```python
from build123d import *

# Parameters (mm, degrees)
F0_W     = 61
F0_H     = 49.2
F1_DEPTH = 1
F2_D     = 3.5
F3_R     = 3.75
F4_DEPTH = 8
F3_R_2   = 6.25
F5_DEPTH = 5
F6_R     = 21
F7_DEPTH = 15
F8_R     = 6.25
F9_DEPTH = 7


with BuildPart() as f1:
    # F0 (on Top) → F1 (new body)
    with BuildSketch(Plane.XY):
        with Locations((30.5, 24.6)):
            Rectangle(F0_W, F0_H)
    extrude(amount=F1_DEPTH)

    # F2 (through all)
    with Locations(Plane(origin=(0, 0, 0), x_dir=(1, 0, 0), z_dir=(0, 0, -1))):
        with Locations((4, -25.5), (57, -25.5)):
            Hole(F2_D / 2)

    # F3 (on face) → F4 (join)
    with BuildSketch(Plane.XY.offset(1)):
        with Locations((30, 21)):
            Circle(F3_R)
    extrude(amount=F4_DEPTH)

    # F3 (on face) → F5 (join)
    with BuildSketch(Plane.XY.offset(1)):
        with BuildLine():
            ThreePointArc((52.5101295887, 49.2), (43.25, 52.7), (33.9898704113, 49.2))
            Line((33.9898704113, 49.2), (52.5101295887, 49.2))
        make_face()
        with BuildLine():
            ThreePointArc((33.9898704113, 49.2), (29.2944841953, 37.5848414357), (35.7748003642, 26.8627118644))
            ThreePointArc((35.7748003642, 26.8627118644), (43.25, 30.5), (50.7251996358, 26.8627118644))
            ThreePointArc((50.7251996358, 26.8627118644), (55.5107665931, 31.9417751924), (57.25, 38.7))
            ThreePointArc((57.25, 38.7), (56.0101295887, 44.4601295887), (52.5101295887, 49.2))
            Line((52.5101295887, 49.2), (33.9898704113, 49.2))
        make_face()
        with Locations((43.25, 38.7)):
            Circle(F3_R_2, mode=Mode.SUBTRACT)
        with Locations((43.25, 38.7)):
            Circle(F3_R_2)
        with BuildLine():
            ThreePointArc((50.7251996358, 26.8627118644), (43.25, 30.5), (35.7748003642, 26.8627118644))
            ThreePointArc((35.7748003642, 26.8627118644), (43.25, 24.7), (50.7251996358, 26.8627118644))
        make_face()
    extrude(amount=F5_DEPTH)

    # F6 (on face) → F7 (join)
    with BuildSketch(Plane.XY):
        with Locations((30, 21)):
            Circle(F6_R)
    extrude(amount=-F7_DEPTH)

    # F8 (on face) → F9 (join)
    with BuildSketch(Plane.XY.offset(6)):
        with Locations((43.25, 38.7)):
            Circle(F8_R)
    extrude(amount=F9_DEPTH)


solid = f1.part
```
Build history of the part. All positions in model axes, mm. A direction names the side the tool comes from. Coordinates: 2 decimals unless noted, no trailing zeros. Order: outer loops, then holes, each group sorted by start corner. A loop starts at its lowest first (then second) coordinate and runs counter-clockwise, first axis right, second up.
Item 1: Drill centre lines: L1, parallel to X at y = 25.5, z = 0.85; L2, parallel to Y at x = 57, z = 0.55; L3, parallel to Z at x = 37.5, y = 2.5. Where is each one in solid material? Low to high.
Filled in:
L1: x = 0 to 2.25, 5.75 to 55.25, 58.75 to 61
L2: y = 0 to 23.75, 27.25 to 49.2
L3: z = -15 to 1
Item 2: Tool access for faces 1 (the flat face through (43, 39, 13)), 2 (the cylindrical face through (29.19, 17.34, 4.94)), 3 (the flat face through (43, 51, 1)), 4 (the flat face through (37, 41, 0)): list every direction of +Z, -Z, +X, -X, +Y, -Y with a clear straight run to the whole face (end or side of a thin tool).
Filled in:
face 1: +Z, +X, -X, +Y, -Y
face 2: +Z
face 3: -Z, +X, -X, +Y
face 4: -Z
Item 3: Saw through at B-B on z = 3.5. List the corners of the cut face in (x, y).
Filled in:
outline: circle Ø7.5 at (30, 21); circle Ø28 at (43.25, 38.7)
Item 4: Drop flat-ended pins along their axis: pin 1 Ø5 at (y, z) = (17, -3) entering from +X; pin 2 Ø4 at (x, y) = (42, 14.5) entering from +Z; pin 3 Ø1.5 at (x, y) = (52.5, 37.5) entering from +Z. Give the stop position or say it passes through.
Filled in:
pin 1: stops at x = 50.95
pin 2: stops at z = 1
pin 3: stops at z = 6
Item 5: Saw through at D-D on y = 35. List the corners of the cut face in (x, z), then the cut area to 3 significant figures.
Filled in:
outline: (0, 0) - (14.35, 0) - (14.35, -15) - (45.65, -15) - (45.65, 0) - (61, 0) - (61, 1) - (56.75, 1) - (56.75, 6) - (48.29, 6) - (48.29, 13) - (38.21, 13) - (38.21, 6) - (29.75, 6) - (29.75, 1) - (0, 1) - close
area: 736 mm2
Item 6: Saw through at A-A on y = 25.5. List the corners of the cut face in (x, z).
Filled in:
outline: (0, 0) - (2.25, 0) - (2.25, 1) - (0, 1) - close; (5.75, 0) - (9.49, 0) - (9.49, -15) - (50.51, -15) - (50.51, 0) - (55.25, 0) - (55.25, 1) - (47.91, 1) - (47.91, 6) - (38.59, 6) - (38.59, 1) - (5.75, 1) - close; (58.75, 0) - (61, 0) - (61, 1) - (58.75, 1) - close
Item 7: Mould opens along X. For faces 5 (the cylindrical face through (46.61, 43.97, 9.45)), 6 (the flat face through (46.2, 32.7, 6)), 7 (the cylindrical face through (55.331, 24.974, 0.507)), 8 (the cylindrical face through (4.228, 23.765, 0.507)) say: released by +X, released by -X, zero draft, split by the parting line, or undercut.
Filled in:
face 5: split by the parting line
face 6: zero draft
face 7: undercut
face 8: undercut
Item 8: Saw through at C-C on x = 54.5. List the corners of the cut face in (y, z).
Filled in:
outline: (0, 0) - (49.2, 0) - (49.2, 1) - (47.03, 1) - (47.03, 6) - (30.37, 6) - (30.37, 1) - (0, 1) - close
